Design review of the part built by this model. Coordinates are the model's own, in mm. Give positions to 0.01 mm unless a question says otherwise; leave off trailing zeros. Order: outer loops, then holes, each group sorted by start corner. A loop starts at its lowest first (then second) coordinate and runs counter-clockwise, first axis right, second up. Notation, with made-up numbers: M 83,21 L 98,21 A10 cw 98,29 Z; hole C -6,6.25 d6. An arc over 180 degrees is marked long. Answer as a JSON object with one key per item and string values.
from build123d import *

# Parameters (mm, degrees)
SKETCH_2_W          = 45
SKETCH_2_H          = 120
SKETCH_2_R          = 2.6
SKETCH_2_R_2        = 1.6
EXTRUDE_1_DEPTH     = 3
SKETCH_3_W          = 17.5
SKETCH_3_H          = 15
CUT_EXTRUDE_1_DEPTH = 3


with BuildPart() as part:
    # 草图2 → 凸台-拉伸1 (new body)
    with BuildSketch(Plane.XY):
        Rectangle(SKETCH_2_W, SKETCH_2_H)
        with Locations((-15, 54)):
            Circle(SKETCH_2_R, mode=Mode.SUBTRACT)
        with Locations((15, 54)):
            Circle(SKETCH_2_R, mode=Mode.SUBTRACT)
        with Locations((0, -41)):
            Circle(SKETCH_2_R_2, mode=Mode.SUBTRACT)
        Polygon((10, 4), (6.535898385, 2), (6.535898385, -2), (10, -4), (13.464101615, -2), (13.464101615, 2), align=None, mode=Mode.SUBTRACT)
        Polygon((0, 4), (-3.464101615, 2), (-3.464101615, -2), (0, -4), (3.464101615, -2), (3.464101615, 2), align=None, mode=Mode.SUBTRACT)
        Polygon((-10, 4), (-13.464101615, 2), (-13.464101615, -2), (-10, -4), (-6.535898385, -2), (-6.535898385, 2), align=None, mode=Mode.SUBTRACT)
        Polygon((10, 14), (6.535898385, 12), (6.535898385, 8), (10, 6), (13.464101615, 8), (13.464101615, 12), align=None, mode=Mode.SUBTRACT)
        Polygon((0, 14), (-3.464101615, 12), (-3.464101615, 8), (0, 6), (3.464101615, 8), (3.464101615, 12), align=None, mode=Mode.SUBTRACT)
        Polygon((-10, 14), (-13.464101615, 12), (-13.464101615, 8), (-10, 6), (-6.535898385, 8), (-6.535898385, 12), align=None, mode=Mode.SUBTRACT)
        Polygon((10, 24), (6.535898385, 22), (6.535898385, 18), (10, 16), (13.464101615, 18), (13.464101615, 22), align=None, mode=Mode.SUBTRACT)
        Polygon((0, 24), (-3.464101615, 22), (-3.464101615, 18), (0, 16), (3.464101615, 18), (3.464101615, 22), align=None, mode=Mode.SUBTRACT)
        Polygon((-10, 24), (-13.464101615, 22), (-13.464101615, 18), (-10, 16), (-6.535898385, 18), (-6.535898385, 22), align=None, mode=Mode.SUBTRACT)
        Polygon((10, 34), (6.535898385, 32), (6.535898385, 28), (10, 26), (13.464101615, 28), (13.464101615, 32), align=None, mode=Mode.SUBTRACT)
        Polygon((0, 34), (-3.464101615, 32), (-3.464101615, 28), (0, 26), (3.464101615, 28), (3.464101615, 32), align=None, mode=Mode.SUBTRACT)
        Polygon((-10, 34), (-13.464101615, 32), (-13.464101615, 28), (-10, 26), (-6.535898385, 28), (-6.535898385, 32), align=None, mode=Mode.SUBTRACT)
        Polygon((10, 44), (6.535898385, 42), (6.535898385, 38), (10, 36), (13.464101615, 38), (13.464101615, 42), align=None, mode=Mode.SUBTRACT)
        Polygon((0, 44), (-3.464101615, 42), (-3.464101615, 38), (0, 36), (3.464101615, 38), (3.464101615, 42), align=None, mode=Mode.SUBTRACT)
        Polygon((-10, 44), (-13.464101615, 42), (-13.464101615, 38), (-10, 36), (-6.535898385, 38), (-6.535898385, 42), align=None, mode=Mode.SUBTRACT)
        Polygon((-10, -6), (-13.464101615, -8), (-13.464101615, -12), (-10, -14), (-6.535898385, -12), (-6.535898385, -8), align=None, mode=Mode.SUBTRACT)
        Polygon((0, -6), (-3.464101615, -8), (-3.464101615, -12), (0, -14), (3.464101615, -12), (3.464101615, -8), align=None, mode=Mode.SUBTRACT)
        Polygon((10, -6), (6.535898385, -8), (6.535898385, -12), (10, -14), (13.464101615, -12), (13.464101615, -8), align=None, mode=Mode.SUBTRACT)
        Polygon((-10, -16), (-13.464101615, -18), (-13.464101615, -22), (-10, -24), (-6.535898385, -22), (-6.535898385, -18), align=None, mode=Mode.SUBTRACT)
        Polygon((0, -16), (-3.464101615, -18), (-3.464101615, -22), (0, -24), (3.464101615, -22), (3.464101615, -18), align=None, mode=Mode.SUBTRACT)
        Polygon((10, -16), (6.535898385, -18), (6.535898385, -22), (10, -24), (13.464101615, -22), (13.464101615, -18), align=None, mode=Mode.SUBTRACT)
        Polygon((-10, -26), (-13.464101615, -28), (-13.464101615, -32), (-10, -34), (-6.535898385, -32), (-6.535898385, -28), align=None, mode=Mode.SUBTRACT)
        Polygon((0, -26), (-3.464101615, -28), (-3.464101615, -32), (0, -34), (3.464101615, -32), (3.464101615, -28), align=None, mode=Mode.SUBTRACT)
        Polygon((10, -26), (6.535898385, -28), (6.535898385, -32), (10, -34), (13.464101615, -32), (13.464101615, -28), align=None, mode=Mode.SUBTRACT)
    extrude(amount=EXTRUDE_1_DEPTH)

    # 草图3 → 切除-拉伸1 (cut)
    with BuildSketch(Plane.XY.offset(3)):
        with Locations((-13.75, -52.5)):
            Rectangle(SKETCH_3_W, SKETCH_3_H)
        with Locations((13.75, -52.5)):
            Rectangle(SKETCH_3_W, SKETCH_3_H)
    extrude(amount=-CUT_EXTRUDE_1_DEPTH, mode=Mode.SUBTRACT)


solid = part.part
(1) We need section B-B (x = 15). Write out the cut boundary in (y, z).
Checked values:
{"outline": "M -45,0 L 51.4,0 L 51.4,3 L -45,3 Z; M 56.6,0 L 60,0 L 60,3 L 56.6,3 Z"}
(2) We need section A-A (y = 54). Write out the cut boundary in (x, z).
Checked values:
{"outline": "M -22.5,0 L -17.6,0 L -17.6,3 L -22.5,3 Z; M -12.4,0 L 12.4,0 L 12.4,3 L -12.4,3 Z; M 17.6,0 L 22.5,0 L 22.5,3 L 17.6,3 Z"}
(3) Insertion check: pin 1 (8 mm diameter, centred on x = 12, y = -16, fed in from -Z); pin 2 (1 mm diameter, centred on x = -7.5, z = 1, fed in from -Y). Each pin has a flat end and moves straight along its axis. Give the tip position at first contact, or say it passes through.
Checked values:
{"pin 1": "stops at z = 0", "pin 2": "stops at y = -45"}
(4) Draft analysis for pull direction X (two halves, no side actions). For faces 1 (the flat face through (-1.708, -6.986, 1.479)), 2 (the flat face through (-5, -53, 2)), 3 (the flat face through (-13.464, -30, 1)), state which applies: +X half, -X half, draft (parallel to the pull), parting line (faces both ways), or undercut.
Checked values:
{"face 1": "undercut", "face 2": "-X half", "face 3": "undercut"}
(5) We need section D-D (z = 1.95). Count the separate pieces of the cut face and the enclosed holes in it, plus the area to 3 significant figures.
Checked values:
{"separate pieces": "1", "enclosed holes": "27", "area": "3,830 mm^2"}
(6) We need section C-C (y = -0.5). Write out the cut boundary in (x, z), plus the area to 3 significant figures.
Checked values:
{"outline": "M -22.5,0 L -13.46,0 L -13.46,3 L -22.5,3 Z; M -6.54,0 L -3.46,0 L -3.46,3 L -6.54,3 Z; M 3.46,0 L 6.54,0 L 6.54,3 L 3.46,3 Z; M 13.46,0 L 22.5,0 L 22.5,3 L 13.46,3 Z", "area": "72.6 mm^2"}
(7) To check wall thickness, follow L1, parallel to X at y = 28.5, z = 0.75; L2, parallel to Y at x = 15, z = 0.9; L3, parallel to X at y = -32.5, z = 2.4. State the ranges of each line that lie inside material, in increasing order. Write a range as from..to.
Checked values:
{"L1": "x = -22.5..-13.46, -6.54..-3.46, 3.46..6.54, 13.46..22.5", "L2": "y = -45..51.4, 56.6..60", "L3": "x = -22.5..-12.6, -7.4..-2.6, 2.6..7.4, 12.6..22.5"}
